Input: part model. Units: mm. Frame: model coordinates. A direction names the side the tool comes from. Round coordinates to 2 decimals unless told otherwise and drop trailing zeros. Order: outer loops, then holes, each group sorted by start corner. A loop starts at its lowest first (then second) coordinate and runs counter-clockwise, first axis right, second up. Notation, with made-up numbers: (78.5, -20) -> (126.5, -20) arc R20 ccw to (126.5, 2) -> close; hole circle Ø9 at (-3.75, -40). An arc over 180 degrees is marked (long way). Use a Markdown table: item, result.
Autodesk Inventor part; units mm, degrees
ref_plane "YZ Plane" through (0, 0, 0) normal (1, 0, 0) x (0, 1, 0)
ref_plane "XZ Plane" through (0, 0, 0) normal (0, 1, 0) x (-1, 0, 0)
ref_plane "XY Plane" through (0, 0, 0) normal (0, 0, 1) x (1, 0, 0)
sketch "Esboço1" plane through (0, 0, 0) normal (0, 0, 1) x (1, 0, 0)
  line L0 (-20, -47.5) -> (20, -47.5)
  line L1 (20, -47.5) -> (20, 47.5)
  line L2 (20, 47.5) -> (-20, 47.5)
  line L3 (-20, 47.5) -> (-20, -47.5)
  line L4 (-20, 47.5) -> (20, 47.5)
  circle A0 centre (0, 37.5) radius 5
  circle A1 centre (0, 37.5) radius 27.5862 construction
  circle A2 centre (0, 37.5) radius 74 construction
  line L5 (-20, 18.5) -> (20, 18.5)
  line L6 (-20, -36.5) -> (20, -36.5)
  line L7 (-103.6, 0) -> (103.6, 0) construction
  line L8 (0, -79.3) -> (0, 143.3) construction
  point P0 (0, 0)
  dimension "d0" = 95
  dimension "d1" = 40
  dimension "d41" = 10
  dimension "d42" = 85
  dimension "d43" = 55.1725
  dimension "d45" = 84
  dimension "d49" = 66
extrude "Extrusão1" add sketch "Esboço1" along normal mid plane 10 contours L3 L6 L1 L0 | L3 L5 L1 L6 | L3 L2 L1 L5 | A0
extrude "Extrusão4" cut sketch "Esboço1" against normal blind 2.5 from surface at 5 contours L3 L5 L1 L6
sketch "Esboço2" plane through (-20, -47.5, -5) normal (0, -1, 0) x (1, 0, 0)
  line L0 (40, 10) -> (40, 0)
  line L1 (40, 5) -> (0, 5) construction
  line L2 (0, 0) -> (0, 10)
  line L3 (0, 0) -> (0, 10)
  line L4 (40, 0) -> (40, 10)
  line L5 (0, 10) -> (40, 10) construction
  line L6 (20, 10) -> (20, 0) construction
  line L7 (40, 0) -> (0, 0) construction
  point P0 (20, 5)
  point P1 (7.5, 5)
  point P2 (32.5, 5)
  dimension "d9" = 7.5
  dimension "d10" = 7.5
  dimension "d37" = 25
hole "Furo1" at (-12.5, -47.5, 0) at (12.5, -47.5, 0) direction (0, 1, 0) diameter 3.242 depth 15 tip angle 118
sketch "Esboço3" plane through (0, 0, 5) normal (0, 0, 1) x (1, 0, 0)
  point P0 (0, 0)
  point P1 (0, 37.5)
  point P2 (0, 37.5)
hole "Furo2" at (0, 37.5, 5) direction (0, 0, -1) diameter 6 end through all counterbore diameter 10 counterbore depth 7
fillet "Arredondamento3" radius 2 4 edges at (-20, 18.5, 3.75) (20, 18.5, 3.75) (-20, -36.5, 3.75) (20, -36.5, 3.75)
chamfer "Chanfro2" distance 2 angle 45 2 edges at (-20, 47.5, 0) (20, 47.5, 0)
properties part number "GRJ-03-114" material "Fenolite OR"
1) Pin query (flat end, axial travel): pin 1 Ø2.5 at (x, z) = (-12.5, 0) entering from -Y; pin 2 Ø20 at (x, y) = (9, -13.5) entering from +Z. Return the tip coordinate at first contact, or that it passes through.
Results found:
| item | result |
|---|---|
| pin 1 | stops at y = -32.28 |
| pin 2 | stops at z = 2.5 |
2) Cut plane D-D on x = -10. Return loops of the section in (y, z).
Results found:
| item | result |
|---|---|
| outline | (-47.5, -5) -> (47.5, -5) -> (47.5, 5) -> (18.5, 5) -> (18.5, 2.5) -> (-36.5, 2.5) -> (-36.5, 5) -> (-47.5, 5) -> close |
3) Cut plane A-A on z = 4. Return loops of the section in (x, y).
Results found:
| item | result |
|---|---|
| outline | (-20, -47.5) -> (20, -47.5) -> (20, -38.5) arc R2 ccw to (18, -36.5) -> (-18, -36.5) arc R2 ccw to (-20, -38.5) -> close; (-20, 20.5) arc R2 ccw to (-18, 18.5) -> (18, 18.5) arc R2 ccw to (20, 20.5) -> (20, 45.5) -> (18, 47.5) -> (-18, 47.5) -> (-20, 45.5) -> close; hole circle Ø10 at (0, 37.5) |
4) Set-up query: faces 4 (the cylindrical face through (19.4, -37.07, 3.73)), 5 (the cylindrical face through (-19.43, -37.1, 3.73)), 6 (the flat face through (0, -36.5, 4)). Return all of +Z, -Z, +X, -X, +Y, -Y with unobstructed straight access to the full face (end or side cutting, diameter ignored); none if empty.
Results found:
| item | result |
|---|---|
| face 4 | +Z, +X |
| face 5 | +Z, -X |
| face 6 | +Z, +X, -X |
5) Cut plane B-B on y = 37.5. Return loops of the section in (x, z), and give its area (3 significant figures).
Results found:
| item | result |
|---|---|
| outline | (-20, -5) -> (-3, -5) -> (-3, -2) -> (-5, -2) -> (-5, 5) -> (-20, 5) -> close; (3, -5) -> (20, -5) -> (20, 5) -> (5, 5) -> (5, -2) -> (3, -2) -> close |
| area | 312 mm² |
6) Pull-direction query (Z, two-part tool) for faces 1 (the flat face through (0, 30, 5)), 2 (the cylindrical face through (19.43, 19.1, 3.73)), 3 (the cylindrical face through (10.893, -39.895, 0.211)); classes: +Z half, -Z half, draft (parallel to the pull), parting line (faces both ways), or undercut.
Results found:
| item | result |
|---|---|
| face 1 | +Z half |
| face 2 | draft |
| face 3 | undercut |
7) Line query: L1, parallel to X at y = -37.25, z = 0; L2, parallel to Y at x = -14, z = 4; L3, parallel to Y at x = 4, z = 4.5. Output: solid intervals per line, ascending. Write a range as [from, to].
Results found:
| item | result |
|---|---|
| L1 | x = [-20, -14.12], [-10.88, 10.88], [14.12, 20] |
| L2 | y = [-47.5, -36.5], [18.5, 47.5] |
| L3 | y = [-47.5, -36.5], [18.5, 34.5], [40.5, 47.5] |
8) Cut plane C-C on x = 0. Return loops of the section in (y, z).
Results found:
| item | result |
|---|---|
| outline | (-47.5, -5) -> (34.5, -5) -> (34.5, -2) -> (32.5, -2) -> (32.5, 5) -> (18.5, 5) -> (18.5, 2.5) -> (-36.5, 2.5) -> (-36.5, 5) -> (-47.5, 5) -> close; (40.5, -5) -> (47.5, -5) -> (47.5, 5) -> (42.5, 5) -> (42.5, -2) -> (40.5, -2) -> close |
